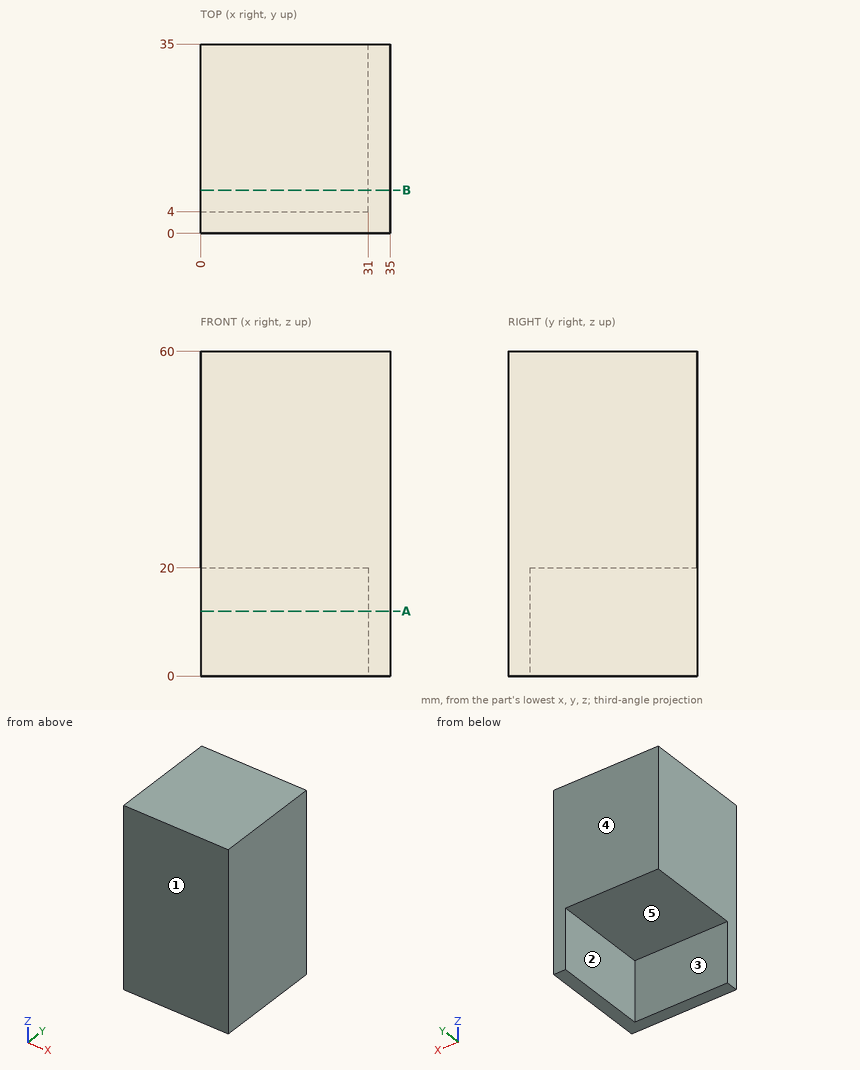
Job drawing, mm, ordinate dimensions from the low corner. One solid piece. A direction names the side the tool comes from. Coordinates: 2 decimals unless noted, no trailing zeros. Write each loop counter-clockwise with the first axis right and the second up, starting at its lowest first coordinate (ties: lowest second). Pieces come first, ordered by that corner, then holes. Notation, with made-up numbers: M -29,15 L -12,15 A27 cw -12,31 Z; hole C -6,54.5 d8. An arc over 180 degrees is marked long. Answer as a JSON object with one key per item and string values. Group by question number.
1) Mould opens along Y. For the marked faces 1, 2 and 3 say: +Y half, -Y half, draft (parallel to the pull), parting line (faces both ways), or undercut.
2) Tool access for the marked faces 4 and 5: list every direction of +Z, -Z, +X, -X, +Y, -Y with a clear straight run to the whole face (end or side of a thin tool).
3) Pin check, flat tips, straight feed: pin 1 Ø6 at (x, y) = (17.5, 29.5) entering from -Z; pin 2 Ø16 at (y, z) = (19.5, 5.5) entering from -X; pin 3 Ø10 at (x, z) = (23, 7) entering from +Y. Stop position of each tip, or through.
4) Saw through at B-B (y = 8). Write the cut outline in (x, z), plus the area to 3 significant figures.
5) Wall check: line 1 (Z direction, x = 6, y = 30.5); line 2 (X direction, y = 28, z = 19); line 3 (Y direction, x = 27.5, z = 14.5). Give the ranges that are in metal, low to high. Write a range as from..to.
6) Saw through at A-A (z = 12). Write the cut outline in (x, y), plus the area to 3 significant figures.
Values follow:
{
 "1": {"face 1": "-Y half", "face 2": "draft", "face 3": "+Y half"},
 "2": {"face 4": "+Z, -Z, +X, -X, +Y", "face 5": "-Z, -X, +Y"},
 "3": {"pin 1": "stops at z = 20", "pin 2": "stops at x = 31", "pin 3": "stops at y = 4"},
 "4": {"outline": "M 0,20 L 31,20 L 31,0 L 35,0 L 35,60 L 0,60 Z", "area": "1,480 mm2"},
 "5": {"line 1": "z = 20..60", "line 2": "x = 31..35", "line 3": "y = 0..4"},
 "6": {"outline": "M 0,0 L 35,0 L 35,35 L 31,35 L 31,4 L 0,4 Z", "area": "264 mm2"}
}
